The listing builds one solid part. Answer for the finished solid, in the listing's coordinates (mm). A direction names the side the tool comes from. Round coordinates to 2 decimals unless told otherwise and drop trailing zeros. Write each loop counter-clockwise with the first axis right and the second up, starting at its lowest first coordinate (ties: lowest second). Pieces come first, ordered by that corner, then holes. Notation, with made-up numbers: (19.25, -19.5) - (78.25, -19.5) arc R33 ccw to (78.25, 13.5) - close; hole circle Ø10 at (-10.5, 75). An arc over 180 degrees is marked (long way). Answer as CSV lines item,"result". Start each with the question number.
Item 1: Straight lines are drawn through the part: line 1 along X through (y, z) = (24, -317); line 2 along Z through (x, y) = (249, 141); line 3 along X through (y, z) = (95, -305.5). For each, find the intervals that lie inside material, in ascending order. Write a range as [from, to].
Item 2: A cutting plane is placed at C-C on z = -267. Determine the outline of the cut face in (x, y), and give its area (3 significant figures).
Item 3: A cutting plane is placed at B-B on x = 261. Determine the outline of the cut face in (y, z).
Item 4: Flat-ended cylindrical pins translate along their axes: pin 1 (12 mm diameter, centred on x = 295, z = -309.5, fed in from -Y); pin 2 (2 mm diameter, centred on x = 265.5, z = -6, fed in from +Y); pin 3 (6 mm diameter, centred on x = 294.5, y = 36, fed in from -Z). Find the tip coordinate at first contact, or state that the pin passes through.
Item 5: For a pull along Z with two mould halves and no side action, classify faces 1 (the flat face through (296, 107, 33.9)), 2 (the flat face through (264, 134, -194.62)), 3 (the flat face through (255.259, 119.437, 11.662)), 4 (the flat face through (264, 134, -306.38)) as pulls with the +Z half, pulls with the -Z half, needs draft (parallel to the pull), parting line crosses it, or undercut.
Item 6: Which of the six approach directions +Z, -Z, +X, -X, +Y, -Y give full straight-line access (tool end or side, diameter ignored) to faces 5 (the flat face through (264, 134, 28.9)), 6 (the flat face through (278, -60, -337)), 7 (the flat face through (283.23, 148.034, -100.098)), 8 (the flat face through (255.259, 119.437, -323.618)), 9 (the flat face through (255.259, 119.437, -100.098))?
Item 7: A cutting plane is placed at A-A on z = -207.5. Determine the outline of the cut face in (x, y).
```python
from build123d import *

# Parameters (mm, degrees)
HEAD_START          = -349.38
HEAD_FLANGE_DEPTH   = 387.28
PRIMARY_START       = -5.1
PRIMARY_1_DEPTH     = 34
PRIMARY_START_2     = -116.86
PRIMARY_3_DEPTH     = 34
PRIMARY_START_3     = -228.62
PRIMARY_5_DEPTH     = 34
PRIMARY_START_4     = -340.38
PRIMARY_7_DEPTH     = 34
COLLECTOR_START     = -343.38
SKETCH6_R           = 30
COLLECTOR_DEPTH     = 377.28
OUTLET_START        = -60
SKETCH7_R           = 26
OUTLET_PIPE_DEPTH   = 166.73776862
OUTLET_START_2      = -72
SKETCH8_R           = 42
OUTLET_FLANGE_DEPTH = 12
OUTLET_START_3      = -73
SKETCH9_R           = 20
OUTLET_BORE_DEPTH   = 169.73776862


with BuildPart() as part:
    # Sketch1 → Head Flange (new body)
    with BuildSketch(Plane.XY.offset(HEAD_START)):
        with BuildLine():
            Line((231.188562109, 129.365185618), (234.724096015, 125.829651712))
            ThreePointArc((234.724096015, 125.829651712), (236.845416358, 124.950972056), (238.966736702, 125.829651712))
            Line((238.966736702, 125.829651712), (277.150502886, 164.013417896))
            ThreePointArc((277.150502886, 164.013417896), (278.029182543, 166.13473824), (277.150502886, 168.256058583))
            Line((277.150502886, 168.256058583), (273.61496898, 171.791592489))
            Line((273.61496898, 171.791592489), (231.188562109, 129.365185618))
        make_face()
    extrude(amount=HEAD_FLANGE_DEPTH)

    # Sketch2 → Primary 1 (add)
    with BuildSketch(Plane.XY.offset(PRIMARY_START)):
        Polygon((266.543901168, 164.720524677), (310.384521602, 120.879904244), (282.100250354, 92.595632996), (238.259629921, 136.43625343), align=None)
    extrude(amount=PRIMARY_1_DEPTH)

    # Sketch3 → Primary 3 (add)
    with BuildSketch(Plane.XY.offset(PRIMARY_START_2)):
        Polygon((266.543901168, 164.720524677), (310.384521602, 120.879904244), (282.100250354, 92.595632996), (238.259629921, 136.43625343), align=None)
    extrude(amount=PRIMARY_3_DEPTH)

    # Sketch4 → Primary 5 (add)
    with BuildSketch(Plane.XY.offset(PRIMARY_START_3)):
        Polygon((266.543901168, 164.720524677), (310.384521602, 120.879904244), (282.100250354, 92.595632996), (238.259629921, 136.43625343), align=None)
    extrude(amount=PRIMARY_5_DEPTH)

    # Sketch5 → Primary 7 (add)
    with BuildSketch(Plane.XY.offset(PRIMARY_START_4)):
        Polygon((266.543901168, 164.720524677), (310.384521602, 120.879904244), (282.100250354, 92.595632996), (238.259629921, 136.43625343), align=None)
    extrude(amount=PRIMARY_7_DEPTH)

    # Sketch6 → Collector (add)
    with BuildSketch(Plane.XY.offset(COLLECTOR_START)):
        with Locations((296.242385978, 106.73776862)):
            Circle(SKETCH6_R)
    extrude(amount=COLLECTOR_DEPTH)

    # Sketch7 → Outlet Pipe (add)
    with BuildSketch(Plane(origin=(0, 0, 0), x_dir=(1, 0, 0), z_dir=(0, 1, 0)).offset(OUTLET_START)):
        with Locations(Location((296.242385978, 317.38, 0), (0, 0, 270))):
            Circle(SKETCH7_R)
    extrude(amount=OUTLET_PIPE_DEPTH)

    # Sketch8 → Outlet Flange (add)
    with BuildSketch(Plane(origin=(0, 0, 0), x_dir=(1, 0, 0), z_dir=(0, 1, 0)).offset(OUTLET_START_2)):
        with Locations(Location((296.242385978, 317.38, 0), (0, 0, 270))):
            Circle(SKETCH8_R)
    extrude(amount=OUTLET_FLANGE_DEPTH)

    # Sketch9 → Outlet Bore (cut)
    with BuildSketch(Plane(origin=(0, 0, 0), x_dir=(1, 0, 0), z_dir=(0, 1, 0)).offset(OUTLET_START_3)):
        with Locations(Location((296.242385978, 317.38, 0), (0, 0, 270))):
            Circle(SKETCH9_R)
    extrude(amount=OUTLET_BORE_DEPTH, mode=Mode.SUBTRACT)


solid = part.part
```
Geometry says:
1,line 1,"x = [270.25, 276.25], [316.24, 322.24]"
1,line 2,"z = [-349.38, 37.9]"
1,line 3,"x = [268.63, 280.15], [312.33, 323.85]"
2,outline,"(231.19, 129.37) - (234.72, 125.83) arc R3 ccw to (238.97, 125.83) - (277.15, 164.01) arc R3 ccw to (277.15, 168.26) - (273.61, 171.79) - close; circle Ø60 at (296.24, 106.74)"
2,area,"3,300 mm^2"
3,outline,"(-72, -340.23) - (-60, -340.23) - (-60, -294.53) - (-72, -294.53) - close; (113.7, -340.38) - (147.86, -340.38) - (147.86, -349.38) - (159.18, -349.38) - (159.18, 37.9) - (147.86, 37.9) - (147.86, 28.9) - (113.7, 28.9) - (113.7, -5.1) - (147.86, -5.1) - (147.86, -82.86) - (113.7, -82.86) - (113.7, -116.86) - (147.86, -116.86) - (147.86, -194.62) - (113.7, -194.62) - (113.7, -228.62) - (147.86, -228.62) - (147.86, -306.38) - (113.7, -306.38) - close"
4,pin 1,"stops at y = 96.74"
4,pin 2,"stops at y = 164.68"
4,pin 3,"stops at z = -343.38"
5,face 1,"pulls with the +Z half"
5,face 2,"undercut"
5,face 3,"needs draft"
5,face 4,"undercut"
6,face 5,"+Z"
6,face 6,"none"
6,face 7,"+Z, -Z, +X"
6,face 8,"+Z, -Z"
6,face 9,"+Z, -Z, -Y"
7,outline,"(231.19, 129.37) - (234.72, 125.83) arc R3 ccw to (238.97, 125.83) - (243.92, 130.78) - (266.29, 108.41) arc R30 ccw (long way) to (294.57, 136.69) - (272.2, 159.06) - (277.15, 164.01) arc R3 ccw to (277.15, 168.26) - (273.61, 171.79) - close"
